from build123d import *

# Parameters (mm, degrees)
F0_W     = 38.1
F0_H     = 38.1
F1_DEPTH = 38.1
F5_DEPTH = 38.1
F7_DEPTH = 38.1
F8_W     = 25.4
F8_H     = 7.62
F9_DEPTH = 38.1


with BuildPart() as f1:
    # F0 (on Front) → F1 (new body)
    with BuildSketch(Plane.XZ):
        with Locations((19.05, 19.05)):
            Rectangle(F0_W, F0_H)
    extrude(amount=F1_DEPTH)

    # F4 (on face) → F5 (cut)
    with BuildSketch(Plane.YZ.offset(38.1)):
        Polygon((-6.35, 38.1), (-31.75, 38.1), (-26.67, 15.875), (-21.59, 28.575), (-16.51, 28.575), (-11.43, 15.875), align=None)
        Polygon((-31.75, 0), (-38.1, 38.1), (-38.1, 0), align=None)
        Polygon((-19.05, 15.875), (-25.4, 0), (-12.7, 0), align=None)
        Polygon((0, 0), (0, 38.1), (-6.35, 0), align=None)
    extrude(amount=-F5_DEPTH, mode=Mode.SUBTRACT)

    # F6 (on offset) → F7 (cut)
    with BuildSketch(Plane.XZ.offset(38.1)):
        Polygon((0, 0), (6.35, 38.1), (0, 38.1), align=None)
        Polygon((25.4, 38.1), (12.7, 38.1), (19.05, 22.225), align=None)
        Polygon((11.43, 22.225), (6.35, 0), (31.75, 0), (26.67, 22.225), (21.59, 9.525), (16.51, 9.525), align=None)
        Polygon((38.1, 38.1), (31.75, 38.1), (37.899472, 0), (38.1, 0), align=None)
    extrude(amount=-F7_DEPTH, mode=Mode.SUBTRACT)

    # F8 (on offset) → F9 (cut)
    with BuildSketch(Plane.XY.offset(38.1)):
        with Locations((25.4, -11.43)):
            Rectangle(F8_W, F8_H)
        with Locations((12.7, -26.67)):
            Rectangle(F8_W, F8_H)
    extrude(amount=-F9_DEPTH, mode=Mode.SUBTRACT)


solid = f1.part
Build history of the part. All positions in model axes, mm. A direction names the side the tool comes from. Give positions to 0.01 mm unless a question says otherwise; leave off trailing zeros. Order: outer loops, then holes, each group sorted by start corner. A loop starts at its lowest first (then second) coordinate and runs counter-clockwise, first axis right, second up. Notation, with made-up numbers: M 70.25,77.5 L 74.25,77.5 A20 cw 74.25,96.5 Z; hole C 35,-20.5 d10. An arc over 180 degrees is marked long. Put each result on its own line as item: value.
Item 1: Which spindle directions (+Z, -Z, +X, -X, +Y, -Y) get a long thin tool onto all of the face, cutting with end or side? Do faces 1 (the face through (3, -9, 0)), 2 (the face through (3.13, -9.05, 18.78)), 3 (the face through (11, -19, 28.575)), 4 (the face through (24.6, -15.24, 18.1)), 5 (the face through (19, -32, 9.525)). Say none if no direction does.
Results are:
face 1: -Z, +X, -X, +Y, -Y
face 2: +Z, -X, +Y, -Y
face 3: +Z, +X, -X
face 4: +Z, -Z, +X
face 5: -Z, +Y, -Y
Item 2: Cut at A-A on z = 7. Write the cut outline in (x, y).
Results are:
outline: M 1.17,-32.92 L 7.95,-32.92 L 7.95,-30.48 L 1.17,-30.48 Z; M 1.17,-22.86 L 7.95,-22.86 L 7.95,-22.6 L 1.17,-22.6 Z; M 1.17,-15.5 L 7.95,-15.5 L 7.95,-5.18 L 1.17,-5.18 Z; M 30.15,-32.92 L 36.77,-32.92 L 36.77,-22.6 L 30.15,-22.6 Z; M 30.15,-15.5 L 36.77,-15.5 L 36.77,-15.24 L 30.15,-15.24 Z; M 30.15,-7.62 L 36.77,-7.62 L 36.77,-5.18 L 30.15,-5.18 Z
Item 3: Pull direction X, two halves, no side cores. Call faces 6 (the face through (10.24, -31.124, 35.361)), 7 (the face through (28.68, -25.49, 13.43)), 8 (the face through (3.836, -33.497, 23.017)): +X half, -X half, draft (parallel to the pull), parting line (faces both ways), or undercut.
Results are:
face 6: draft
face 7: undercut
face 8: -X half
Item 4: Cut at B-B on x = 15.5. Write the cut outline in (y, z) (3 decimals), then the cut area to 3 significant figures.
Results are:
outline: M -36.933,31.1 L -33.758,12.05 L -30.48,12.05 L -30.48,31.1 Z; M -22.86,12.05 L -20.58,12.05 L -19.05,15.875 L -17.52,12.05 L -15.24,12.05 L -15.24,25.4 L -16.51,28.575 L -21.59,28.575 L -22.86,25.4 Z; M -7.62,12.05 L -4.342,12.05 L -1.167,31.1 L -7.62,31.1 Z
area: 301 mm2
Item 5: Cut at D-D on z = 14. Count the separate pieces of the cut face and the enclosed holes in it, then the cut area to 3 significant figures.
Results are:
separate pieces: 10
enclosed holes: 0
area: 415 mm2
Item 6: Wall check: probe 1 along X at (y, z) = (-4, 15); probe 2 along Y at (x, z) = (10, 17); probe 3 along X at (y, z) = (-33, 15.5). Give the ranges that are in metal, low to high.
Results are:
probe 1: 2.5 to 9.78, 14.32 to 23.78, 28.32 to 35.48
probe 2: -34.58 to -30.48, -22.86 to -11.88, -11.17 to -3.52
probe 3: 2.58 to 9.89, 14.12 to 23.98, 28.21 to 35.4
Item 7: Drop flat-ended pins along their axis: pin 1 Ø1 at (x, y) = (13, -22) entering from +Z (3 decimals); pin 2 Ø10 at (y, z) = (-10.5, 24.5) entering from +X; pin 3 Ø3.5 at (y, z) = (-29.5, 23) entering from -X. Give the stop position or say it passes through.
Results are:
pin 1: z = 28.575
pin 2: x = 34.6
pin 3: x = 3.59
